Here's the drawing with two shaded views (mm, measured from the low corner). I have some questions. Coordinates: 2 decimals unless noted, no trailing zeros. Loops run counter-clockwise (first coordinate to the right, second up) from the corner with the lowest first, then second, coordinate; pieces in that order, holes last. Notation, with made-up numbers: (11.5, 79) -> (36.5, 79) arc R7 ccw to (36.5, 91) -> close; hole circle Ø5 at (-12, 76.25). An arc over 180 degrees is marked (long way). Answer as a JSON object with one key per item and string values. Group by question number.
Q1. I want a section at B-B on y = 0.65. Write out the boundary of the cut face in (x, z), then the cut area to 3 significant figures.
Q2. I want a section at D-D on x = 6.35. Write out the boundary of the cut face in (y, z).
Q3. I need wall thicknesses on line 1 (Z direction, x = 6.35, y = 0.65); line 2 (X direction, y = 0.4, z = 35.5); line 3 (Z direction, x = 27, y = 0.55) (1 decimal). Which ranges of each line are inside material? Lowest first, please.
Q4. I want a section at C-C on x = 35.56. Write out the boundary of the cut face in (y, z).
Q5. I want a section at A-A on z = 35.56. Write out the boundary of the cut face in (x, y).
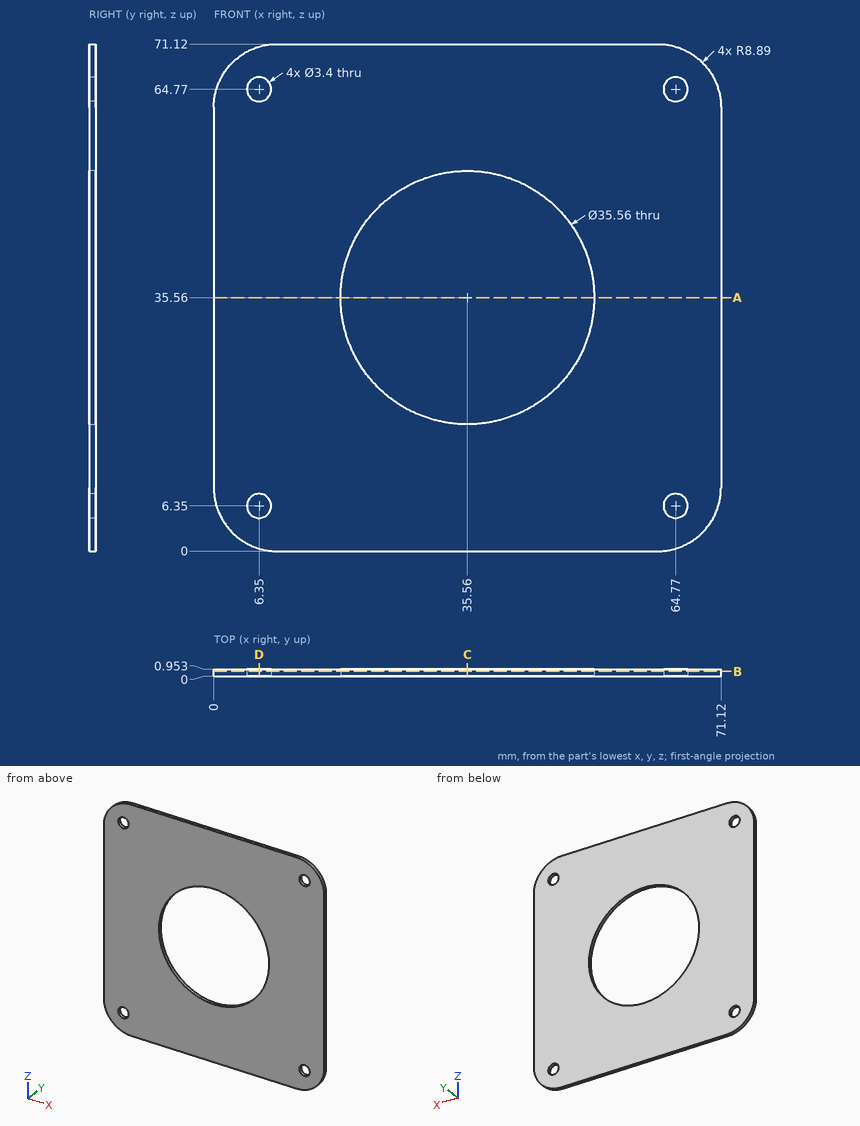
Result set:
{
 "1": {"outline": "(0, 8.89) arc R8.89 ccw to (8.89, 0) -> (62.23, 0) arc R8.89 ccw to (71.12, 8.89) -> (71.12, 62.23) arc R8.89 ccw to (62.23, 71.12) -> (8.89, 71.12) arc R8.89 ccw to (0, 62.23) -> close; hole circle Ø3.4 at (6.35, 6.35); hole circle Ø3.4 at (6.35, 64.77); hole circle Ø35.56 at (35.56, 35.56); hole circle Ø3.4 at (64.77, 6.35); hole circle Ø3.4 at (64.77, 64.77)", "area": "3,960 mm²"},
 "2": {"outline": "(0, 0.37) -> (0.95, 0.37) -> (0.95, 4.65) -> (0, 4.65) -> close; (0, 8.05) -> (0.95, 8.05) -> (0.95, 63.07) -> (0, 63.07) -> close; (0, 66.47) -> (0.95, 66.47) -> (0.95, 70.75) -> (0, 70.75) -> close"},
 "3": {"line 1": "z = 0.37 to 4.65, 8.05 to 63.07, 66.47 to 70.75", "line 2": "x = 0 to 17.78, 53.34 to 71.12", "line 3": "z = 0 to 20, 51.1 to 71.1"},
 "4": {"outline": "(0, 0) -> (0.95, 0) -> (0.95, 17.78) -> (0, 17.78) -> close; (0, 53.34) -> (0.95, 53.34) -> (0.95, 71.12) -> (0, 71.12) -> close"},
 "5": {"outline": "(0, 0) -> (17.78, 0) -> (17.78, 0.95) -> (0, 0.95) -> close; (53.34, 0) -> (71.12, 0) -> (71.12, 0.95) -> (53.34, 0.95) -> close"}
}
